Source: CAD feature listing. Evaluate the final solid. Frame: model axes, mm. A direction names the side the tool comes from. Give positions to 0.01 mm unless a question says otherwise; leave off trailing zeros. Order: outer loops, then holes, each group sorted by start corner. A loop starts at its lowest first (then second) coordinate and runs counter-clockwise, first axis right, second up. Notation, with made-up numbers: M 32.25,-31.75 L 41.25,-31.75 A22 ccw 41.25,-25.75 Z; hole C 59,53 d4. An arc over 180 degrees is marked long. Use CSV: the item, a comma, the result in double quotes. Start each with the question number.
Item 1: Access query for faces 1 (the face through (0, 0, -16.65)), 2 (the face through (0, 9.75, 50)), 3 (the face through (0, 7, 56.97)), 4 (the face through (0, 4, 49)), 5 (the face through (13.6, -12.2, 16.65)). Directions: +Z, -Z, +X, -X, +Y, -Y. A direction counts if a zero-diameter tool reaches every point of the face in a straight line with its end or side. Return the directions, or none.
Item 2: First-contact query: pin 1 (10 mm diameter, centred on x = 13.5, z = 22, fed in from +Y); pin 2 (2 mm diameter, centred on x = 14.5, y = 2.5, fed in from +Z); pin 3 (3 mm diameter, centred on x = 5.5, z = 3.5, fed in from +Y). Flat tips, straight axial feed; report the tip coordinate or a pass-through.
Item 3: Section query B-B on y = 0. Return loops of the section in (x, z), and give its area (3 significant figures).
Item 4: Section query A-A on x = 0. Return loops of the section in (y, z).
Item 5: Section query C-C on z = 40. Return loops of the section in (x, y).
Item 6: Ray query, probe 1 along Z at (x, y) = (8.5, 7); probe 2 along Z at (x, y) = (10, 15.5); probe 3 along Y at (x, z) = (0, 5.5). Return the intervals inside material, ascending. Write a range as from..to.
Item 7: Section query D-D on y = 7. Return loops of the section in (x, z), and give its area (3 significant figures).
from build123d import *

# Parameters (mm, degrees)
SKETCH1_R           = 18.1
BOSS_EXTRUDE1_DEPTH = 16.65
SKETCH2_R           = 18.5
BOSS_EXTRUDE2_DEPTH = 20.32
SKETCH3_R           = 5.999999938
BOSS_EXTRUDE3_DEPTH = 5
SKETCH4_R           = 3
BOSS_EXTRUDE4_DEPTH = 15
SKETCH5_W           = 2.397915762
SKETCH5_H           = 1.769215018
CUT_EXTRUDE1_DEPTH  = 15


with BuildPart() as part:
    # Sketch1 → Boss-Extrude1 (new, symmetric)
    with BuildSketch(Plane.XY):
        Circle(SKETCH1_R)
    extrude(amount=BOSS_EXTRUDE1_DEPTH, both=True)

    # Sketch2 → Boss-Extrude2 (add)
    with BuildSketch(Plane.XY.offset(16.65)):
        Circle(SKETCH2_R)
    extrude(amount=BOSS_EXTRUDE2_DEPTH)

    # Sketch3 → Boss-Extrude3 (add)
    with BuildSketch(Plane.XY.offset(36.97)):
        with Locations((0, 7)):
            Circle(SKETCH3_R)
    extrude(amount=BOSS_EXTRUDE3_DEPTH)

    # Sketch4 → Boss-Extrude4 (add)
    with BuildSketch(Plane.XY.offset(41.97)):
        with Locations((0, 7)):
            Circle(SKETCH4_R)
    extrude(amount=BOSS_EXTRUDE4_DEPTH)

    # Sketch5 → Cut-Extrude1 (cut)
    with BuildSketch(Plane.XY.offset(56.97)):
        with Locations((0, 10.634607509)):
            Rectangle(SKETCH5_W, SKETCH5_H)
    extrude(amount=-CUT_EXTRUDE1_DEPTH, mode=Mode.SUBTRACT)


solid = part.part
Verdict:
1,face 1,"-Z, +X, -X, +Y, -Y"
1,face 2,"+Z, +X, -X, +Y"
1,face 3,"+Z, +X, -X, +Y, -Y"
1,face 4,"+Z"
1,face 5,"-Z"
2,pin 1,"y = 16.43"
2,pin 2,"z = 36.97"
2,pin 3,"y = 17.65"
3,outline,"M -18.5,16.65 L -18.1,16.65 L -18.1,-16.65 L 18.1,-16.65 L 18.1,16.65 L 18.5,16.65 L 18.5,36.97 L -18.5,36.97 Z"
3,area,"1,960 mm2"
4,outline,"M -18.5,16.65 L -18.1,16.65 L -18.1,-16.65 L 18.1,-16.65 L 18.1,16.65 L 18.5,16.65 L 18.5,36.97 L 13,36.97 L 13,41.97 L 9.75,41.97 L 9.75,56.97 L 4,56.97 L 4,41.97 L 1,41.97 L 1,36.97 L -18.5,36.97 Z"
5,outline,"C 0,7 d12"
6,probe 1,"-16.65..36.97"
6,probe 2,"16.65..36.97"
6,probe 3,"-18.1..18.1"
7,outline,"M -17.12,16.65 L -16.69,16.65 L -16.69,-16.65 L 16.69,-16.65 L 16.69,16.65 L 17.12,16.65 L 17.12,36.97 L 6,36.97 L 6,41.97 L 3,41.97 L 3,56.97 L -3,56.97 L -3,41.97 L -6,41.97 L -6,36.97 L -17.12,36.97 Z"
7,area,"1,960 mm2"
